Study the drawing (mm; zero at the part's minimum x, y, z) and answer. Round coordinates to 2 decimals unless told otherwise and drop trailing zeros. Write each loop counter-clockwise with the first axis right and the second up, starting at its lowest first coordinate (ties: lowest second). Pieces come first, ordered by that corner, then holes.
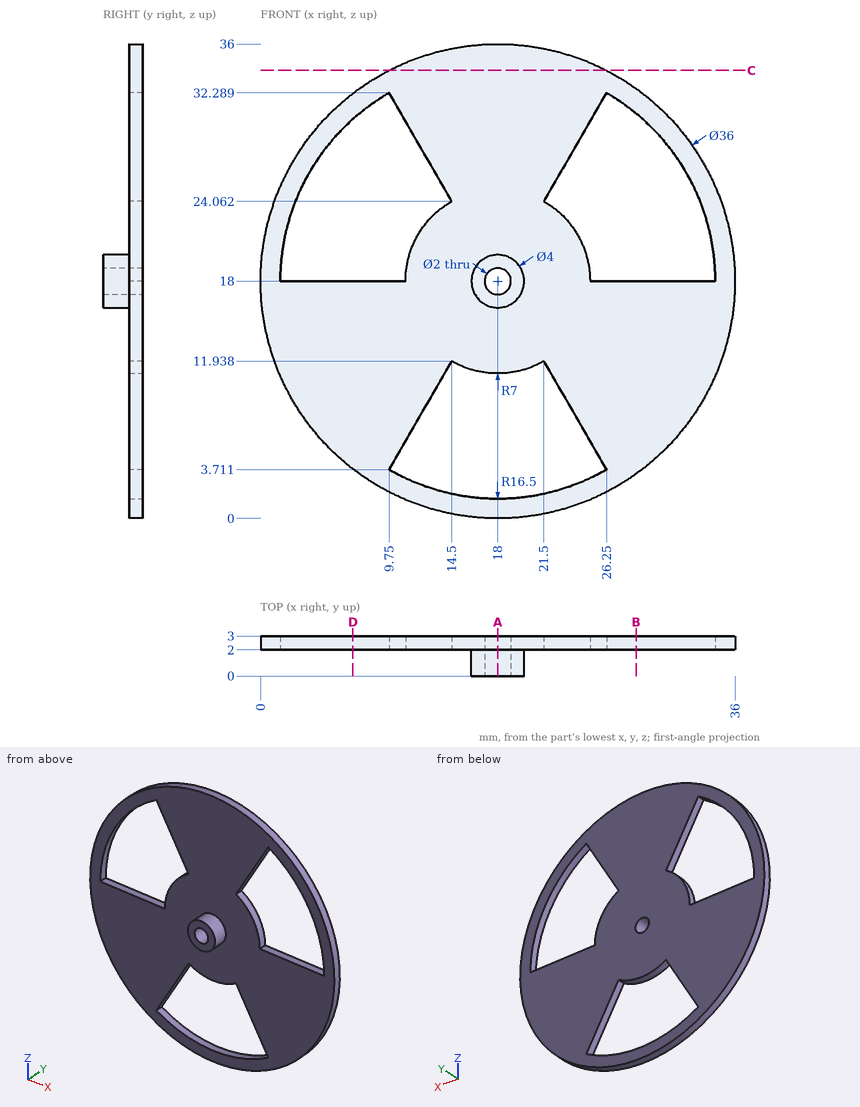
Q1. Given pin 1 (4 mm diameter, centred on x = 30.5, z = 3.5, fed in from -Y); pin 2 (0.8 mm diameter, centred on x = 8.5, y = 2.5, fed in from +Z); pin 3 (1 mm diameter, centred on y = 2, z = 17, fed in from -X), each flat-ended and moving along its own axis, determine where each tip first touches the part or whether it passes through.
Q2. Find the intervals of material crossed by L1, parallel to X at y = 0.15, z = 18; L2, parallel to Z at x = 13, y = 2.85 (1 decimal); L3, parallel to X at y = 2.2, z = 31.5 (1 decimal), in increasing order.
Q3. Find section A-A (x = 18). Determine the outline of the cut face in (y, z).
Q4. Find section B-B (x = 28.5). Determine the outline of the cut face in (y, z), plus the area to 3 significant figures.
Q5. Find section D-D (x = 7). Determine the outline of the cut face in (y, z).
Q6. Find section C-C (z = 34). Determine the outline of the cut face in (x, y), plus the area to 3 significant figures.
Report:
1. pin 1: stops at y = 2
1. pin 2: stops at z = 33.53
1. pin 3: stops at x = 0.01
2. L1: x = 16 to 17, 19 to 20
2. L2: z = 0.7 to 2.3, 9.3 to 22.9, 26.7 to 35.3
2. L3: x = 6.1 to 8.5, 10.2 to 25.8, 27.5 to 29.9
3. outline: (0, 16) - (2, 16) - (2, 11) - (3, 11) - (3, 17) - (0, 17) - close; (0, 19) - (3, 19) - (3, 36) - (2, 36) - (2, 20) - (0, 20) - close; (2, 0) - (3, 0) - (3, 1.5) - (2, 1.5) - close
4. outline: (2, 3.38) - (3, 3.38) - (3, 18) - (2, 18) - close; (2, 30.73) - (3, 30.73) - (3, 32.62) - (2, 32.62) - close
4. area: 16.5 mm2
5. outline: (2, 3.75) - (3, 3.75) - (3, 18) - (2, 18) - close; (2, 30.3) - (3, 30.3) - (3, 32.25) - (2, 32.25) - close
6. outline: (9.75, 2) - (26.25, 2) - (26.25, 3) - (9.75, 3) - close
6. area: 16.5 mm2
